```python
from build123d import *

# Parameters (mm, degrees)
F0_W      = 228.6
F0_H      = 228.6
F1_DEPTH  = 19.05
F3_DEPTH  = 19.051
F5_DEPTH  = 63.5
F7_W      = 77.47
F7_H      = 7.62
F8_DEPTH  = 33.02
F6_W      = 161.6446101792
F6_H      = 19.05
F6_W_2    = 76.2
F6_H_2    = 6.35
F9_DEPTH  = 31.75
F11_W     = 33.95681642
F11_H     = 16.0381817259
F12_ANGLE = 35


with BuildPart() as f1:
    # F0 (on Top) → F1 (new body)
    with BuildSketch(Plane.XY):
        with Locations((4.8490930349, 10.9562167545)):
            Rectangle(F0_W, F0_H)
    extrude(amount=F1_DEPTH)

    # F2 (on face) → F3 (cut, through all)
    with BuildSketch(Plane.XY.offset(19.05)):
        Polygon((155.7185798883, -103.3437832455), (119.1490930349, 125.2562167545), (-109.4509069651, -103.3437832455), align=None)
    extrude(amount=-F3_DEPTH, mode=Mode.SUBTRACT)

    # F4 (on face) → F5 (cut, symmetric)
    with BuildSketch(Plane.XY.offset(19.05)):
        Polygon((150.6341397762, 139.1298025846), (-109.4509069651, 125.2562167545), (4.8490930349, 10.9562167545), align=None)
    extrude(amount=F5_DEPTH, both=True, mode=Mode.SUBTRACT)

    # F7 (on face) → F8 (cut)
    with BuildSketch(Plane(origin=(-3.0535618598, 3.0535618598, 0), x_dir=(0.7071067812, 0.7071067812, 0), z_dir=(0.7071067812, -0.7071067812, 0))):
        with Locations((-74.9035684484, 3.81)):
            Rectangle(F7_W, F7_H)
    extrude(amount=-F8_DEPTH, mode=Mode.SUBTRACT)

    # F6 (on face) → F9 (join)
    with BuildSketch(Plane(origin=(7.9026548947, 7.9026548947, 0), x_dir=(-0.7071067812, 0.7071067812, 0), z_dir=(0.7071067812, 0.7071067812, 0))):
        with Locations((85.1406936854, 9.525)):
            Rectangle(F6_W, F6_H)
        with Locations((89.8955209156, 6.35)):
            Rectangle(F6_W_2, F6_H_2, mode=Mode.SUBTRACT)
    extrude(amount=F9_DEPTH)

    # F11 (on 3pt) → F12 (revolve, cut)
    with BuildSketch(Plane(origin=(-40.1975363097, 22.1779510674, 0), x_dir=(-0.4830773429, -0.875577684, 0), z_dir=(-0.875577684, 0.4830773429, 0))):
        with Locations((41.3631814837, -0.3990908629)):
            Rectangle(F11_W, F11_H)
    revolve(axis=Axis((-109.4509069651, -103.3437832455, 9.525), (0, 0, -1)), revolution_arc=F12_ANGLE, mode=Mode.SUBTRACT)


solid = f1.part
```
Model file for the job. Use its own axes, mm. A direction names the side the tool comes from. Give positions to 0.01 mm unless a question says otherwise; leave off trailing zeros. Order: outer loops, then holes, each group sorted by start corner. A loop starts at its lowest first (then second) coordinate and runs counter-clockwise, first axis right, second up.
1) Saw through at C-C, the plane x = -36. Write the cut outline in (y, z) (3 decimals), then the cut area to 3 significant figures.
2) Saw through at B-B, the plane y = 116. Write the cut outline in (x, z) (3 decimals).
3) Pin check, flat tips, straight feed: pin 1 (2 mm diameter, centred on y = 64, z = 10.5, fed in from +X); pin 2 (3 mm diameter, centred on x = -72, z = 11, fed in from -Y); pin 3 (5 mm diameter, centred on y = 122.5, z = 3.5, fed in from +X). Stop position of each tip, or through.
4) 3-axis set-ups, long thin cutter, end or side, ignore diameter. For faces 4 (the cylindrical face through (-38.132, -8.116, 3.863)), 5 (the flat face through (-71.536, 109.477, 6.306)), 6 (the flat face through (-94.92, -65.79, 3.76)), 7 (the flat face through (-44, 82, 3.175)), 8 (the flat face through (-67, -39, 7.62)): which of +Z, -Z, +X, -X, +Y, -Y reach the whole face in a straight line?
5) Saw through at A-A, the plane x = -77.5. Write the cut outline in (y, z) (3 decimals).
6) Saw through at D-D, the plane z = 15.5. Write the cut outline in (x, y).
7) Wall check: probe 1 along Z at (x, y) = (-26, 80) (3 decimals); probe 2 along Z at (x, y) = (-41, -24.5); probe 3 along X at (y, z) = (-49, 7.25). Give the ranges that are in metal, low to high.
8) Mould opens along X. For faces 1 (the flat face through (-70, 23, 19.05)), 2 (the flat face through (-98.383, 136.324, 9.392)), 3 (the flat face through (-56.04, 71.846, 6.394)) say: +X half, -X half, draft (parallel to the pull), parting line (faces both ways), or undercut.
Computed:
1. outline: (-29.893, 7.62) - (-9.75, 7.62) - (-9.75, 0) - (96.707, 0) - (96.707, 3.175) - (51.805, 3.175) - (51.805, 9.525) - (96.707, 9.525) - (96.707, 19.05) - (-29.893, 19.05) - close
1. area: 1,970 mm2
2. outline: (-109.451, 0) - (-55.293, 0) - (-55.293, 3.175) - (-65.013, 3.175) - (-65.013, 9.525) - (-55.293, 9.525) - (-55.293, 19.05) - (-109.451, 19.05) - close
3. pin 1: stops at x = -2.29
3. pin 2: stops at y = -67.39
3. pin 3: stops at x = -59.31
4. face 4: -Z, -Y
4. face 5: +X
4. face 6: -Z, +X
4. face 7: none
4. face 8: -Z
5. outline: (-71.393, 7.62) - (-24.696, 7.62) - (-24.696, 0) - (138.207, 0) - (138.207, 19.05) - (-71.393, 19.05) - close; hole (93.305, 3.175) - (103.513, 3.175) - (103.513, 9.525) - (93.305, 9.525) - close
6. outline: (-109.45, -103.34) - (27.3, 33.41) - (-87, 147.71) - (-109.45, 125.26) - close
7. probe 1: z = 0 to 3.175, 9.525 to 19.05
7. probe 2: z = 7.62 to 19.05
7. probe 3: x = -109.45 to -101.8
8. face 1: draft
8. face 2: -X half
8. face 3: undercut
